```python
from build123d import *

# Parameters (mm, degrees)
SKETCH1_R           = 25
SKETCH1_R_2         = 5
BOSS_EXTRUDE1_DEPTH = 5
CUT_EXTRUDE1_DEPTH  = 10


with BuildPart() as part:
    # Sketch1 → Boss-Extrude1 (new body, symmetric)
    with BuildSketch(Plane.XY):
        Circle(SKETCH1_R)
        Circle(SKETCH1_R_2, mode=Mode.SUBTRACT)
    extrude(amount=BOSS_EXTRUDE1_DEPTH, both=True)

    # Sketch2 → Cut-Revolve1 (revolve, cut)
    with BuildSketch(Plane(origin=(0, 0, 0), x_dir=(0, 0, -1), z_dir=(1, 0, 0))):
        Polygon((-2.5, 27), (-1.25, 23), (1.25, 23), (2.5, 27), align=None)
    revolve(axis=Axis((0, 0, 14.237449017), (0, 0, -1)), mode=Mode.SUBTRACT)

    # Sketch3 → Cut-Extrude1 (cut)
    with BuildSketch(Plane(origin=(0, 0, -5), x_dir=(-1, 0, 0), z_dir=(0, 0, -1))):
        with BuildLine():
            Line((-1.732878986, 6.690109852), (1.732878986, 6.690109852))
            Line((1.732878986, 6.690109852), (1.732878986, 4.690109852))
            ThreePointArc((1.732878986, 4.690109852), (0, 5), (-1.732878986, 4.690109852))
            Line((-1.732878986, 4.690109852), (-1.732878986, 6.690109852))
        make_face()
    extrude(amount=-CUT_EXTRUDE1_DEPTH, mode=Mode.SUBTRACT)


solid = part.part
```
Source: CAD feature listing. Evaluate the final solid. Frame: model axes, mm. A direction names the side the tool comes from. Round coordinates to 2 decimals unless told otherwise and drop trailing zeros. Loops run counter-clockwise (first coordinate to the right, second up) from the corner with the lowest first, then second, coordinate; pieces in that order, holes last. Notation, with made-up numbers: M -22.5,-10 L 22.5,-10 A20 cw 22.5,21 Z; hole C -34,1 d1. An arc over 180 degrees is marked long. Use a Markdown table: item, result. Add a question column.
1. Line query: line 1 (X direction, y = 0, z = 3); line 2 (X direction, y = 2, z = 0); line 3 (Y direction, x = 2, z = 3.75). Output: solid intervals per line, ascending.
2. Mould query, pull axis Z, two halves, no side actions, for faces 1 (the flat face through (0, 6.69, 0)), 2 (the flat face through (-0.3, -5.2, 5)), 3 (the cylindrical face through (22.804, -2.994, -0.018)). Classes: pulls with the +Z half, pulls with the -Z half, needs draft (parallel to the pull), parting line crosses it, or undercut.
3. Section query A-A on y = 0. Return the cut outline in (x, z) (3 decimals), then the cut area to 4 significant figures.
4. Section query B-B on x = 0. Return the cut outline in (y, z) (3 decimals), then the cut area to 3 significant figures.
5. Section query D-D on z = 3.25. Return the cut outline in (x, y).
6. Contact query for flat-ended pins moving along their axis: P1, Ø6, axis at x = -19, z = 0, coming from the +Y side; P2, Ø1, axis at x = -18.5, z = -2.5, coming from the -Y side; P3, Ø3, axis at x = 2, z = -0.5, coming from the -Y side; P4, Ø16, axis at x = 0, y = 0, coming from the +Z side. Output: stop coordinate, or through.
7. Reachability of faces 4 (the flat face through (-0.3, -5.2, -5)), 5 (the flat face through (1.733, 6, 0)) from +Z, -Z, +X, -X, +Y, -Y: full face, straight path, thin tool, end or side. Return the list, or none.
8. Section query C-C on z = 0.5. Return the cut outline in (x, y), then the cut area to 3 significant figures.
Reported:
| question | item | result |
|---|---|---|
| 1 | line 1 | x = -25 to -5, 5 to 25 |
| 1 | line 2 | x = -22.91 to -4.58, 4.58 to 22.91 |
| 1 | line 3 | y = -24.92 to -4.58, 4.58 to 24.92 |
| 2 | face 1 | needs draft |
| 2 | face 2 | pulls with the +Z half |
| 2 | face 3 | undercut |
| 3 | outline | M -25,-5 L -5,-5 L -5,5 L -25,5 L -25,1.875 L -23,1.25 L -23,-1.25 L -25,-1.875 Z; M 5,-5 L 25,-5 L 25,-1.875 L 23,-1.25 L 23,1.25 L 25,1.875 L 25,5 L 5,5 Z |
| 3 | area | 387.5 mm² |
| 4 | outline | M -25,-5 L -5,-5 L -5,5 L -25,5 L -25,1.875 L -23,1.25 L -23,-1.25 L -25,-1.875 Z; M 6.69,-5 L 25,-5 L 25,-1.875 L 23,-1.25 L 23,1.25 L 25,1.875 L 25,5 L 6.69,5 Z |
| 4 | area | 371 mm² |
| 5 | outline | C 0,0 d50; hole M -1.73,4.69 A5 ccw long 1.73,4.69 L 1.73,6.69 L -1.73,6.69 Z |
| 6 | P1 | stops at y = 18.64 |
| 6 | P2 | stops at y = -17.35 |
| 6 | P3 | stops at y = -24.96 |
| 6 | P4 | stops at z = 5 |
| 7 | face 4 | -Z, +X, -X, +Y, -Y |
| 7 | face 5 | +Z, -Z |
| 8 | outline | C 0,0 d46; hole M -1.73,4.69 A5 ccw long 1.73,4.69 L 1.73,6.69 L -1.73,6.69 Z |
| 8 | area | 1,580 mm² |
